```python
from build123d import *

# Parameters (mm, degrees)
BOSS_EXTRUDE1_DEPTH = 2.5
SKETCH4_R           = 1.78
CUT_EXTRUDE1_DEPTH  = 1.5
FILLET1_R           = 1.5


with BuildPart() as part:
    # Sketch2 → Boss-Extrude1 (new body)
    with BuildSketch(Plane(origin=(0, 0, 0), x_dir=(1, 0, 0), z_dir=(0, 1, 0))):
        Polygon((-21.216153836, 11.741903429), (-21.216153836, 8.241903429), (-12.024866066, -0.958096571), (4.783846164, -0.958096571), (12.783846164, 3.741903429), (12.783846164, 11.741903429), align=None)
    extrude(amount=BOSS_EXTRUDE1_DEPTH)

    # Sketch4 → Cut-Extrude1 (cut)
    with BuildSketch(Plane(origin=(0, 2.5, 0), x_dir=(1, 0, 0), z_dir=(0, 1, 0))):
        with Locations((-17.966153836, 8.241903429)):
            Circle(SKETCH4_R)
        with Locations((9.533846164, 8.241903429)):
            Circle(SKETCH4_R)
    extrude(amount=-CUT_EXTRUDE1_DEPTH, mode=Mode.SUBTRACT)

    # Fillet1
    fillet1_edges = [part.edges().sort_by_distance(p)[0] for p in [
        (12.783846164, 1.25, -11.741903429),
        (12.783846164, 1.25, -3.741903429),
        (4.783846164, 1.25, 0.958096571),
        (-12.024866066, 1.25, 0.958096571),
        (-21.216153836, 1.25, -8.241903429),
        (-21.216153836, 1.25, -11.741903429),
        (12.783846164, 0, -7.741903429),
        (8.783846164, 0, -1.391903429),
        (-3.620509951, 0, 0.958096571),
        (-16.620509951, 0, -3.641903429),
        (-21.216153836, 0, -9.991903429),
        (-4.216153836, 0, -11.741903429),
    ]]
    fillet(fillet1_edges, radius=FILLET1_R)


solid = part.part
```
Source: CAD feature listing. Evaluate the final solid. Frame: model axes, mm. A direction names the side the tool comes from. Give positions to 0.01 mm unless a question says otherwise; leave off trailing zeros. Write each loop counter-clockwise with the first axis right and the second up, starting at its lowest first coordinate (ties: lowest second). Pieces come first, ordered by that corner, then holes. Notation, with made-up numbers: (52.5, 75.25) - (60.5, 75.25) arc R20 cw to (60.5, 84.25) - close; hole circle Ø6 at (-34, 32). An arc over 180 degrees is marked (long way). One line per item, written item: value. Start each with the question number.
Q1. Draft query along Z for faces 3 (the face through (12.333, 0.428, -7.461)), 4 (the face through (8.22, 1.76, -9.44)), 5 (the face through (-21.105, 2.007, -8.297)), 6 (the face through (-4.433, 0.451, -11.314)). Return one class per face: +Z half, -Z half, draft (parallel to the pull), parting line (faces both ways), or undercut.
Q2. Material intervals for probe 1 along X at (y, z) = (1.45, -9); probe 2 along X at (y, z) = (1.95, -7); probe 3 along Y at (x, z) = (9.5, -8.75), sorted ascending. Write a range as from..to.
Q3. First-contact query: pin 1 Ø2 at (x, z) = (9.53, -8.24) entering from +Y. Flat tip, straight axial feed; report the tip coordinate or a pass-through.
Q4. Section query A-A, the plane x = -11. Return the cut outline in (y, z), then the cut area to 3 significant figures.
Q5. Set-up query: faces 1 (the face through (-18, 1, -8)), 2 (the face through (-4, 2, -11.742)). Return all of +Z, -Z, +X, -X, +Y, -Y with unobstructed straight access to the full face (end or side cutting, diameter ignored); none if empty.
Answer:
1. face 3: draft
1. face 4: undercut
1. face 5: +Z half
1. face 6: -Z half
2. probe 1: x = -21.22..-19.58, -16.36..7.92, 11.14..12.78
2. probe 2: x = -19.98..-19.24, -16.69..8.26, 10.81..12.78
2. probe 3: y = 0..1
3. pin 1: stops at y = 1
4. outline: (0, -10.24) arc R1.5 ccw to (1.5, -11.74) - (2.5, -11.74) - (2.5, 0.96) - (1.5, 0.96) arc R1.5 ccw to (0, -0.54) - close
4. area: 30.8 mm2
5. face 1: +Y
5. face 2: -Z, +X, -X, +Y, -Y
